For this review, use the dimensioned drawing (mm, ordinates from the lowest corner) and the shaded views. A direction names the side the tool comes from. Give positions to 0.01 mm unless a question says otherwise; leave off trailing zeros. Write each loop counter-clockwise with the first axis right and the second up, starting at its lowest first coordinate (ties: lowest second). Pieces come first, ordered by that corner, then holes. Notation, with made-up numbers: M 32,-13.75 L 91,-13.75 A28 ccw 91,12.25 Z; hole C 62,29.5 d6. An arc over 180 degrees is marked long. Answer in a Markdown table with one row per item.
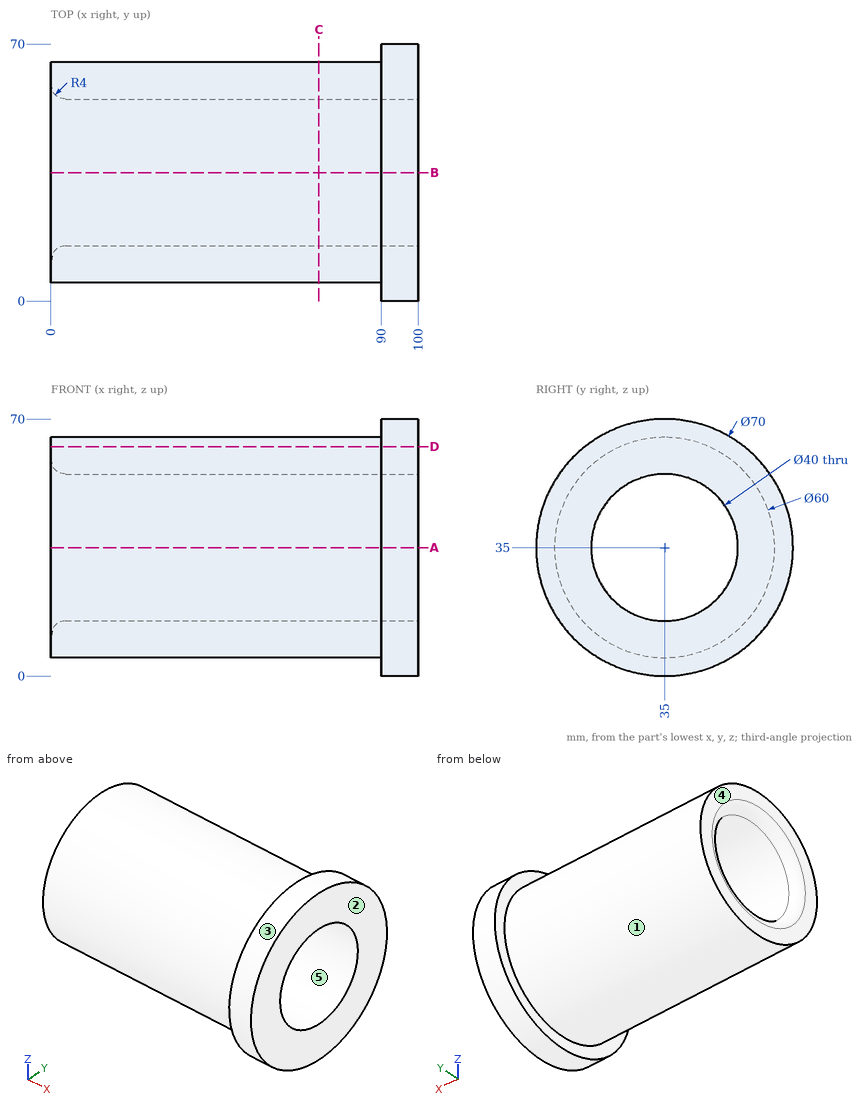
1) The part is to be moulded in two halves that separate along Z. For the marked faces 3, 4 and 5, say which applies: released by +Z, released by -Z, zero draft, split by the parting line, or undercut.
Geometry says:
| item | result |
|---|---|
| face 3 | split by the parting line |
| face 4 | zero draft |
| face 5 | undercut |
2) Add section C-C (x = 73). Write out the cut boundary in (y, z).
Geometry says:
| item | result |
|---|---|
| outline | C 35,35 d60; hole C 35,35 d40 |
3) For the marked faces 1 and 2, list the 3-axis set-ups (+Z, -Z, +X, -X, +Y, -Y) from which the entire face can be reached by the end or side of a thin tool; tool diameter is ignored.
Geometry says:
| item | result |
|---|---|
| face 1 | -X |
| face 2 | +Z, -Z, +X, +Y, -Y |
4) Insertion check: P1, Ø10, axis at x = 79.5, z = 51.5, coming from the -Y side; P2, Ø24, axis at y = 35, z = 35, coming from the -X side; P3, Ø1.5, axis at x = 77.5, y = 17, coming from the -Z side; P4, Ø6, axis at x = 58, y = 58.5, coming from the +Z side. Each pin has a flat end and moves straight along its axis. Give the tip position at first contact, or say it passes through.
Geometry says:
| item | result |
|---|---|
| P1 | y = 7.29 |
| P2 | through |
| P3 | z = 10.46 |
| P4 | z = 56.9 |
5) To check wall thickness, follow probe 1 along Y at (x, z) = (46, 35); probe 2 along Z at (x, y) = (10, 34.5); probe 3 along Z at (x, y) = (11, 29). State the ranges of each line that lie inside material, in increasing order. Write a range as [from, to].
Geometry says:
| item | result |
|---|---|
| probe 1 | [5, 15], [55, 65] |
| probe 2 | [5, 15.01], [54.99, 65] |
| probe 3 | [5.61, 15.92], [54.08, 64.39] |
6) Add section D-D (z = 62.5). Write out the cut boundary in (x, y).
Geometry says:
| item | result |
|---|---|
| outline | M 0,23.01 L 90,23.01 L 90,13.35 L 100,13.35 L 100,56.65 L 90,56.65 L 90,46.99 L 0,46.99 Z |
7) Add section A-A (z = 35). Write out the cut boundary in (x, y), and give its area (3 significant figures).
Geometry says:
| item | result |
|---|---|
| outline | M 0,5 L 90,5 L 90,0 L 100,0 L 100,15 L 4,15 A4 ccw 0,11 Z; M 0,59 A4 ccw 4,55 L 100,55 L 100,70 L 90,70 L 90,65 L 0,65 Z |
| area | 2,090 mm^2 |
